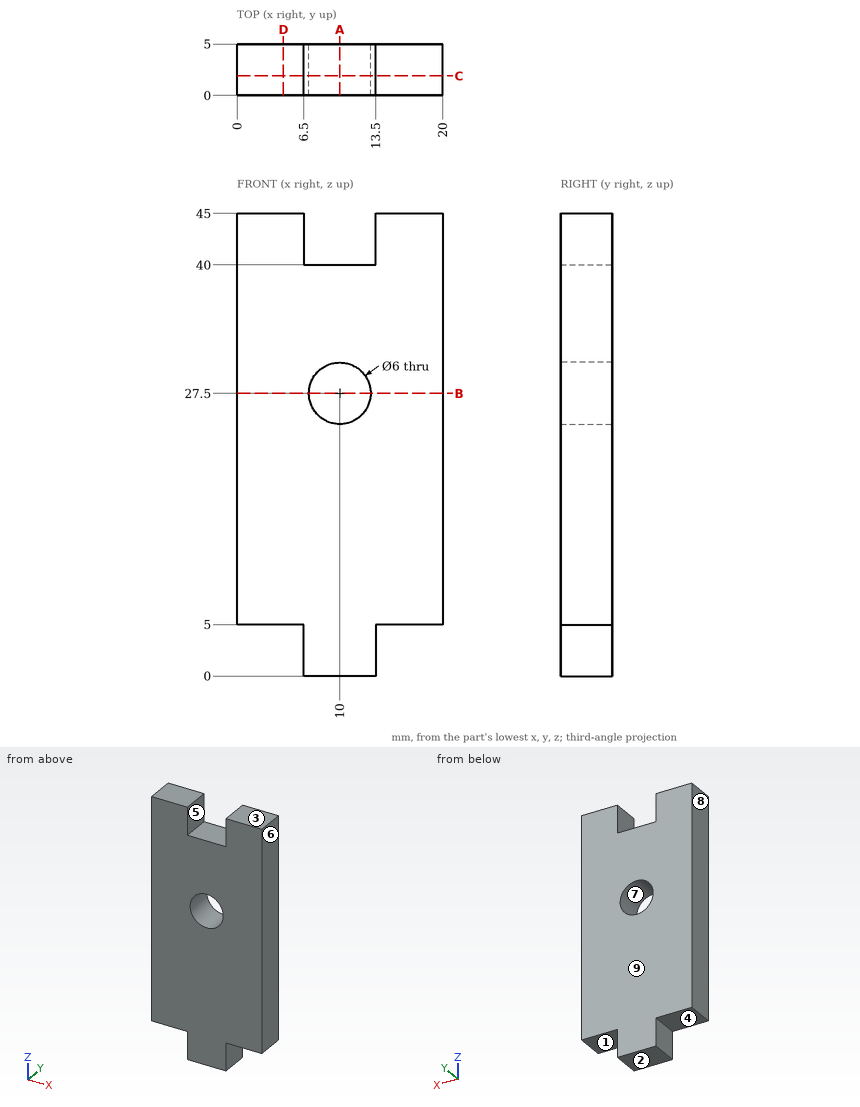
Source: three-view drawing plus pictorial views. Frame: mm from the lowest corner of the part. A direction names the side the tool comes from. Coordinates: 2 decimals unless noted, no trailing zeros. Write each loop counter-clockwise with the first axis right and the second up, starting at its lowest first coordinate (ties: lowest second). Pieces come first, ordered by that corner, then holes. Notation, with made-up numbers: (-18.5, -17.5) - (-0.5, -17.5) arc R30 cw to (-0.5, 6.5) - close; hole circle Ø3 at (-27, -27). An arc over 180 degrees is marked (long way). Answer as a JSON object with one key per item and string values.
Q1. Section query D-D, the plane x = 4.5. Output: boundary loops of the cut face in (y, z), plus the area to 3 significant figures.
Ans:
{"outline": "(0, 5) - (5, 5) - (5, 45) - (0, 45) - close", "area": "200 mm2"}
Q2. Section query A-A, the plane x = 10. Output: boundary loops of the cut face in (y, z), plus the area to 3 significant figures.
Ans:
{"outline": "(0, 0) - (5, 0) - (5, 24.5) - (0, 24.5) - close; (0, 30.5) - (5, 30.5) - (5, 40) - (0, 40) - close", "area": "170 mm2"}
Q3. Section query B-B, the plane z = 27.5. Output: boundary loops of the cut face in (x, y), plus the area to 3 significant figures.
Ans:
{"outline": "(0, 0) - (7, 0) - (7, 5) - (0, 5) - close; (13, 0) - (20, 0) - (20, 5) - (13, 5) - close", "area": "70.0 mm2"}
Q4. Material intervals for line 1 (X direction, y = 3.45, z = 27.5); line 2 (X direction, y = 4.85, z = 3.5); line 3 (Z direction, x = 10.5, y = 2.95), sorted ascending. Write a range as [from, to].
Ans:
{"line 1": "x = [0, 7], [13, 20]", "line 2": "x = [6.5, 13.5]", "line 3": "z = [0, 24.54], [30.46, 40]"}
Q5. Section query C-C, the plane y = 1.9. Output: boundary loops of the cut face in (x, z), plus the area to 3 significant figures.
Ans:
{"outline": "(0, 5) - (6.5, 5) - (6.5, 0) - (13.5, 0) - (13.5, 5) - (20, 5) - (20, 45) - (13.5, 45) - (13.5, 40) - (6.5, 40) - (6.5, 45) - (0, 45) - close; hole circle Ø6 at (10, 27.5)", "area": "772 mm2"}
Q6. First-contact query: pin 1 Ø2.5 at (x, y) = (2, 2) entering from -Z; pin 2 Ø2.5 at (y, z) = (3.5, 41.5) entering from -X; pin 3 Ø2.5 at (y, z) = (3.5, 3.5) entering from -X; pin 4 Ø5 at (x, z) = (10, 27.5) entering from -Y (3 decimals). Flat tips, straight axial feed; report the tip coordinate or a pass-through.
Ans:
{"pin 1": "stops at z = 5", "pin 2": "stops at x = 0", "pin 3": "stops at x = 6.5", "pin 4": "passes through"}
Q7. Draft query along X for the marked faces 6, 7, 8 and 9. Return one class per face: released by +X, released by -X, zero draft, split by the parting line, or undercut.
Ans:
{"face 6": "released by +X", "face 7": "undercut", "face 8": "released by -X", "face 9": "zero draft"}
Q8. Set-up query: the marked faces 1, 2, 3, 4 and 5. Return all of +Z, -Z, +X, -X, +Y, -Y with unobstructed straight access to the full face (end or side cutting, diameter ignored); none if empty.
Ans:
{"face 1": "-Z, +X, +Y, -Y", "face 2": "-Z, +X, -X, +Y, -Y", "face 3": "+Z, +X, -X, +Y, -Y", "face 4": "-Z, -X, +Y, -Y", "face 5": "+Z, +Y, -Y"}
